Geometry: see drawing. Coordinates: mm, zero at the bounding-box minimum. A direction names the side the tool comes from. Coordinates: 2 decimals unless noted, no trailing zeros. Write each loop counter-clockwise with the first axis right and the second up, starting at its lowest first coordinate (ties: lowest second). Pieces come first, ordered by that corner, then holes. Notation, with made-up numbers: (73.25, -27) - (124.25, -27) arc R18 cw to (124.25, -10) - close; hole circle Ø11 at (65, -19). An arc over 180 degrees is marked (long way). Use a Markdown table: item, result. Add a question column.
Q1. Set-up query: the marked faces 1, 2 and 3. Return all of +Z, -Z, +X, -X, +Y, -Y with unobstructed straight access to the full face (end or side cutting, diameter ignored); none if empty.
Q2. Section query B-B (y = 80). Return the cut outline in (x, z), then the cut area to 3 significant figures.
Q3. Mould query, pull axis Z, two halves, no side actions, for the marked faces 4, 5 and 6. Classes: released by +Z, released by -Z, zero draft, split by the parting line, or undercut.
Q4. Section query A-A (z = 74). Return the cut outline in (x, y), then the cut area to 3 significant figures.
Q5. Material intervals for probe 1 along Z at (x, y) = (156.25, 6); probe 2 along Y at (x, z) = (18.25, 14.5); probe 3 along Z at (x, y) = (8.5, 145.5), sorted ascending. Write a range as from..to.
Q6. Section query D-D (y = 139). Return the cut outline in (x, z), then the cut area to 3 significant figures.
Q7. Section query C-C (x = 119.5). Return the cut outline in (y, z).
Q8. Pin query (flat end, axial travel): P1, Ø3, axis at x = 46, z = 141.5, coming from the -Y side; P2, Ø16.5, axis at x = 159.5, z = 113.5, coming from the +Y side; P3, Ø4, axis at x = 18.25, y = 176.75, coming from the -Z side; P4, Ø3, axis at x = 18.25, y = 133.25, coming from the -Z side. Return the tip coordinate at first contact, or that it passes through.
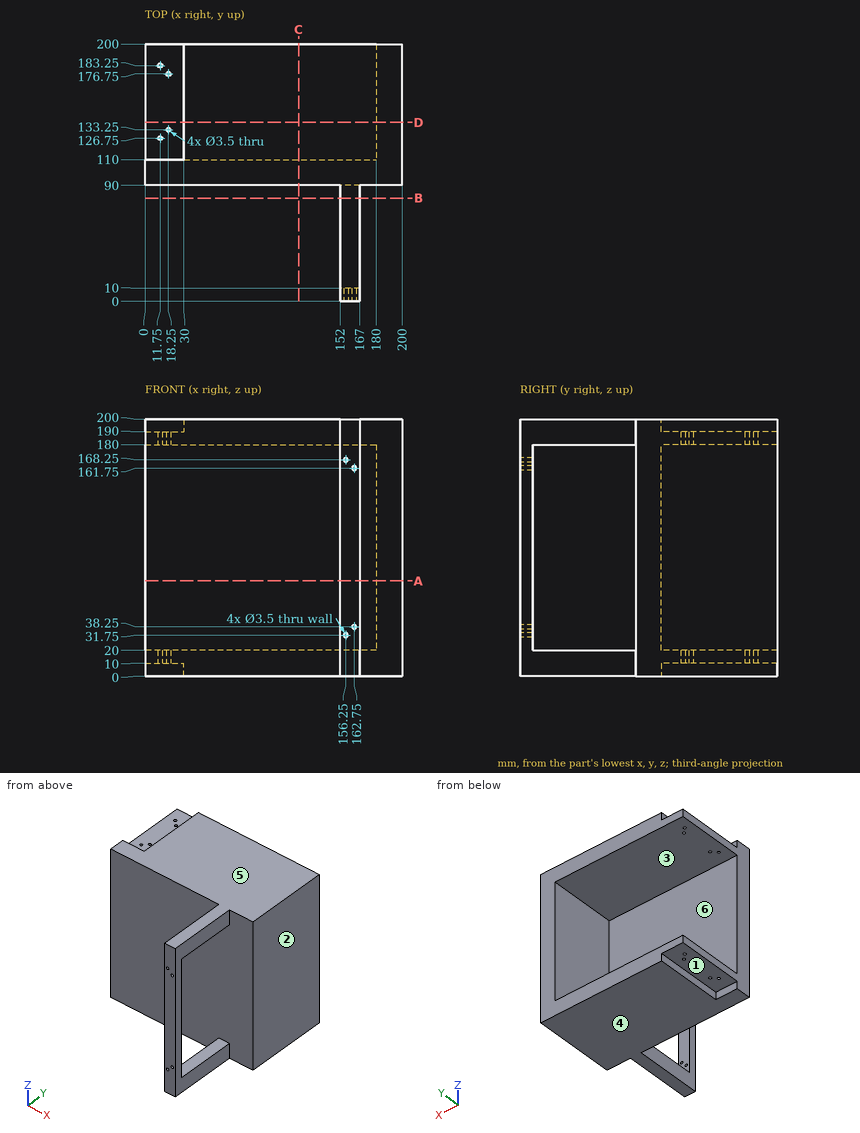
Values follow:
| question | item | result |
|---|---|---|
| 1 | face 1 | -Z, -X, +Y |
| 1 | face 2 | +Z, -Z, +X, +Y, -Y |
| 1 | face 3 | -X, +Y |
| 2 | outline | (152, 0) - (167, 0) - (167, 20) - (152, 20) - close; (152, 180) - (167, 180) - (167, 200) - (152, 200) - close |
| 2 | area | 600 mm2 |
| 3 | face 4 | released by -Z |
| 3 | face 5 | released by +Z |
| 3 | face 6 | undercut |
| 4 | outline | (0, 90) - (200, 90) - (200, 200) - (180, 200) - (180, 110) - (0, 110) - close; (152, 0) - (167, 0) - (167, 10) - (152, 10) - close |
| 4 | area | 5,950 mm2 |
| 5 | probe 1 | 0..30, 33.5..166.5, 170..200 |
| 5 | probe 2 | 90..131.5, 135..175, 178.5..200 |
| 5 | probe 3 | 10..20, 180..190 |
| 6 | outline | (0, 10) - (30, 10) - (30, 0) - (200, 0) - (200, 200) - (30, 200) - (30, 190) - (0, 190) - (0, 180) - (180, 180) - (180, 20) - (0, 20) - close |
| 6 | area | 10,600 mm2 |
| 7 | outline | (90, 0) - (200, 0) - (200, 20) - (110, 20) - (110, 180) - (200, 180) - (200, 200) - (90, 200) - close |
| 8 | P1 | y = 90 |
| 8 | P2 | y = 110 |
| 8 | P3 | z = 10 |
| 8 | P4 | through |
